Here's how the part is built. I have some questions about the finished solid (model axes, mm). A direction names the side the tool comes from. Coordinates: 2 decimals unless noted, no trailing zeros. Loops run counter-clockwise (first coordinate to the right, second up) from the corner with the lowest first, then second, coordinate; pieces in that order, holes last. Notation, with made-up numbers: M 17.5,-17.5 L 53.5,-17.5 A19 ccw 53.5,15.5 Z; hole C 1,84 d1. An arc over 180 degrees is marked long. Use CSV: the item, a comma, the result in double quotes. Start each with the question number.
Q1. If we mould it in two halves opening along X, with no side actions, what happens to faces 1 (the flat face through (42.05, 13, 0)), 2 (the flat face through (48.05, 10, 0)), 3 (the flat face through (1, 10, -33.219))? For each: +X half, -X half, draft (parallel to the pull), parting line (faces both ways), or undercut.
Q2. If we section it at B-B (z = 13): Please give me the cut outline in (x, y).
Q3. For pin 1 Ø6 at (x, z) = (-21, 19) entering from +Y, with a flat end and sliding along its axis, tell me the tip position at first contact or that it passes through.
Q4. Please list where these lines run through material, in increasing order: probe 1 along Z at (x, y) = (0.5, 16.5); probe 2 along X at (y, z) = (7.75, -5); probe 3 along Y at (x, z) = (-0.5, 4.5). Write a range as [from, to].
Q5. If we section it at A-A (y = 13): Please give me the cut outline in (x, z), and give its area (3 significant figures).
Q6. If we section it at C-C (x = -13.5): Please give me the cut outline in (y, z).
Q7. Which directions (+Z, -Z, +X, -X, +Y, -Y) give clear straight access to the entire face, cutting with the end or side of a thin tool? Please do faces 4 (the flat face through (-1, 13, 28.219)), 5 (the flat face through (-48.05, 10, 0)).
from build123d import *

# Parameters (mm, degrees)
SKETCH1_W           = 97.6
SKETCH1_H           = 66.43745389
BOSS_EXTRUDE1_DEPTH = 6
SKETCH4_W           = 24.6
SKETCH4_H           = 54
SKETCH4_H_2         = 6.218726945
SKETCH4_W_2         = 55
SKETCH4_W_3         = 18
BOSS_EXTRUDE2_DEPTH = 13.5
SKETCH6_W           = 97.6
SKETCH6_H           = 56.43745389
CUT_EXTRUDE2_DEPTH  = 13.5
SKETCH7_W           = 66.43745389
SKETCH7_H           = 19.5
CUT_EXTRUDE3_DEPTH  = 0.75
SKETCH8_W           = 66.43745389
SKETCH8_H           = 19.5
CUT_EXTRUDE4_DEPTH  = 0.75
SKETCH9_W           = 6
SKETCH9_H           = 56.43745389
BOSS_EXTRUDE3_DEPTH = 13.5


with BuildPart() as part:
    # Sketch1 → Boss-Extrude1 (new body)
    with BuildSketch(Plane(origin=(0, 0, 0), x_dir=(1, 0, 0), z_dir=(0, 1, 0))):
        Rectangle(SKETCH1_W, SKETCH1_H)
    extrude(amount=BOSS_EXTRUDE1_DEPTH)

    # Sketch4 → Boss-Extrude2 (add)
    with BuildSketch(Plane(origin=(0, 6, 0), x_dir=(1, 0, 0), z_dir=(0, 1, 0))):
        with Locations((-36.5, 0)):
            Rectangle(SKETCH4_W, SKETCH4_H)
        with Locations((-36.5, -30.109363473)):
            Rectangle(SKETCH4_W, SKETCH4_H_2)
        with Locations((3.3, -30.109363473)):
            Rectangle(SKETCH4_W_2, SKETCH4_H_2)
        with Locations((39.8, -30.109363473)):
            Rectangle(SKETCH4_W_3, SKETCH4_H_2)
        with Locations((39.8, 0)):
            Rectangle(SKETCH4_W_3, SKETCH4_H)
        with Locations((39.8, 30.109363473)):
            Rectangle(SKETCH4_W_3, SKETCH4_H_2)
        with Locations((-36.5, 30.109363473)):
            Rectangle(SKETCH4_W, SKETCH4_H_2)
        with Locations((3.3, 30.109363473)):
            Rectangle(SKETCH4_W_2, SKETCH4_H_2)
    extrude(amount=BOSS_EXTRUDE2_DEPTH)

    # Sketch6 → Cut-Extrude2 (cut)
    with BuildSketch(Plane(origin=(0, 19.5, 0), x_dir=(1, 0, 0), z_dir=(0, 1, 0))):
        Rectangle(SKETCH6_W, SKETCH6_H)
    extrude(amount=-CUT_EXTRUDE2_DEPTH, mode=Mode.SUBTRACT)

    # Sketch7 → Cut-Extrude3 (cut)
    with BuildSketch(Plane(origin=(48.8, 0, 0), x_dir=(0, 0, -1), z_dir=(1, 0, 0))):
        with Locations((0, 9.75)):
            Rectangle(SKETCH7_W, SKETCH7_H)
    extrude(amount=-CUT_EXTRUDE3_DEPTH, mode=Mode.SUBTRACT)

    # Sketch8 → Cut-Extrude4 (cut)
    with BuildSketch(Plane.ZY.offset(48.8)):
        with Locations((0, 9.75)):
            Rectangle(SKETCH8_W, SKETCH8_H)
    extrude(amount=-CUT_EXTRUDE4_DEPTH, mode=Mode.SUBTRACT)

    # Sketch9 → Boss-Extrude3 (add)
    with BuildSketch(Plane(origin=(0, 6, 0), x_dir=(1, 0, 0), z_dir=(0, 1, 0))):
        with Locations((-45.05, 0)):
            Rectangle(SKETCH9_W, SKETCH9_H)
        with Locations((45.05, 0)):
            Rectangle(SKETCH9_W, SKETCH9_H)
    extrude(amount=BOSS_EXTRUDE3_DEPTH)


solid = part.part
Results below:
1,face 1,"undercut"
1,face 2,"+X half"
1,face 3,"draft"
2,outline,"M -48.05,0 L 48.05,0 L 48.05,19.5 L 42.05,19.5 L 42.05,6 L -42.05,6 L -42.05,19.5 L -48.05,19.5 Z"
3,pin 1,"y = 6"
4,probe 1,"[-33.22, -28.22], [28.22, 33.22]"
4,probe 2,"[-48.05, -42.05], [42.05, 48.05]"
4,probe 3,"[0, 6]"
5,outline,"M -48.05,-33.22 L 48.05,-33.22 L 48.05,33.22 L -48.05,33.22 Z; hole M -42.05,-28.22 L 42.05,-28.22 L 42.05,28.22 L -42.05,28.22 Z"
5,area,"1,640 mm^2"
6,outline,"M 0,-33.22 L 19.5,-33.22 L 19.5,-28.22 L 6,-28.22 L 6,28.22 L 19.5,28.22 L 19.5,33.22 L 0,33.22 Z"
7,face 4,"+Y"
7,face 5,"+Z, -Z, -X, +Y, -Y"
